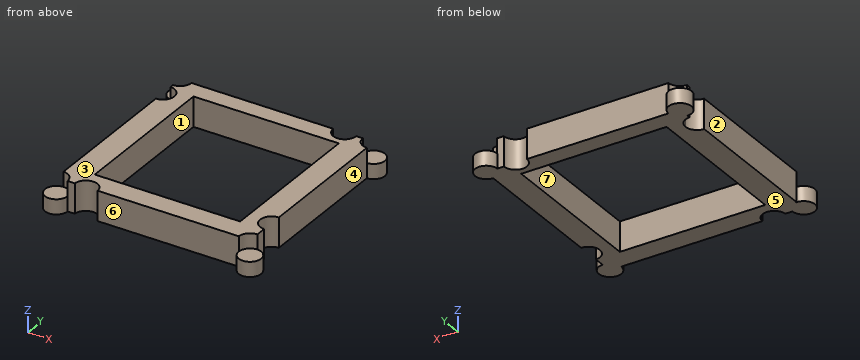
```python
from build123d import *

# Parameters (mm, degrees)
F0_W     = 130.696968
F0_H     = 130.696968
F1_DEPTH = 20
F3_DEPTH = 20
F4_W     = 97.922124
F4_H     = 104.10668
F5_DEPTH = 25
F6_R     = 7.559223
F6_R_2   = 7.71768
F7_DEPTH = 10


with BuildPart() as f1:
    # F0 (on Top) → F1 (new body)
    with BuildSketch(Plane.XY):
        Rectangle(F0_W, F0_H)
    extrude(amount=F1_DEPTH)

    # F2 (on Top) → F3 (cut)
    with BuildSketch(Plane.XY):
        with BuildLine():
            Line((65.463071, -65.384018), (65.463071, -73.302153))
            ThreePointArc((65.463071, -73.302153), (70.877053, -70.99904), (73.111326, -65.556288))
            ThreePointArc((73.111326, -65.556288), (65.450978, -57.810279), (57.620266, -65.384018))
            Line((57.620266, -65.384018), (65.463071, -65.384018))
        make_face()
        with BuildLine():
            ThreePointArc((65.266604, -73.302153), (65.364838, -73.302776), (65.463071, -73.302153))
            Line((65.463071, -73.302153), (65.266604, -73.302153))
        make_face()
        with BuildLine():
            Line((-43.278281, -73.302153), (65.266604, -73.302153))
            ThreePointArc((65.266604, -73.302153), (59.79244, -70.937409), (57.620266, -65.384018))
            Line((57.620266, -65.384018), (-37.424044, -65.384018))
            ThreePointArc((-37.424044, -65.384018), (-37.416151, -65.585784), (-37.413519, -65.787688))
            ThreePointArc((-37.413519, -65.787688), (-39.053255, -70.553782), (-43.278281, -73.302153))
        make_face()
        with BuildLine():
            ThreePointArc((-47.041733, -73.302153), (-45.160007, -73.534176), (-43.278281, -73.302153))
            Line((-43.278281, -73.302153), (-47.041733, -73.302153))
        make_face()
        with BuildLine():
            Line((-52.89597, -65.384018), (-37.424044, -65.384018))
            ThreePointArc((-37.424044, -65.384018), (-45.160007, -58.0412), (-52.89597, -65.384018))
        make_face()
        with BuildLine():
            Line((-52.89597, -73.302153), (-47.041733, -73.302153))
            ThreePointArc((-47.041733, -73.302153), (-51.140461, -70.711329), (-52.89597, -66.191358))
            Line((-52.89597, -66.191358), (-52.89597, -73.302153))
        make_face()
        with BuildLine():
            Line((-52.89597, -66.191358), (-52.89597, -65.384018))
            ThreePointArc((-52.89597, -65.384018), (-52.906495, -65.787688), (-52.89597, -66.191358))
        make_face()
        with BuildLine():
            ThreePointArc((-73.248961, -65.359679), (-65.60328, -73.302152), (-57.75848, -65.556288))
            ThreePointArc((-57.75848, -65.556288), (-60.027374, -60.078694), (-65.504968, -57.8098))
            Line((-65.504968, -57.8098), (-65.504968, -65.365049))
            Line((-65.504968, -65.365049), (-73.248961, -65.365049))
            Line((-73.248961, -65.365049), (-73.248961, -65.359679))
        make_face()
        with BuildLine():
            ThreePointArc((-73.248961, -65.359679), (-70.912604, -60.009617), (-65.504968, -57.8098))
            Line((-65.504968, -57.8098), (-65.504968, 39.620381))
            ThreePointArc((-65.504968, 39.620381), (-70.912604, 41.820198), (-73.248961, 47.17026))
            Line((-73.248961, 47.17026), (-73.248961, -65.359679))
        make_face()
        with BuildLine():
            Line((-65.504968, 54.955278), (-65.504968, 39.620381))
            ThreePointArc((-65.504968, 39.620381), (-60.027374, 41.889275), (-57.75848, 47.366869))
            ThreePointArc((-57.75848, 47.366869), (-60.608689, 53.369745), (-67.061929, 54.955278))
            Line((-67.061929, 54.955278), (-65.504968, 54.955278))
        make_face()
        with BuildLine():
            ThreePointArc((-73.248961, 47.563477), (-73.251456, 47.366869), (-73.248961, 47.17026))
            Line((-73.248961, 47.17026), (-73.248961, 47.563477))
        make_face()
        with BuildLine():
            Line((-73.248961, 54.955278), (-73.248961, 47.563477))
            ThreePointArc((-73.248961, 47.563477), (-71.445222, 52.338937), (-67.061929, 54.955278))
            Line((-67.061929, 54.955278), (-73.248961, 54.955278))
        make_face()
        with BuildLine():
            ThreePointArc((-64.895208, 73.134162), (-71.194062, 60.154116), (-57.75848, 65.411709))
            Line((-57.75848, 65.411709), (-65.504968, 65.411709))
            Line((-65.504968, 65.411709), (-65.504968, 73.134162))
            Line((-65.504968, 73.134162), (-64.895208, 73.134162))
        make_face()
        with BuildLine():
            ThreePointArc((-64.895208, 73.134162), (-59.815874, 70.669303), (-57.75848, 65.411709))
            Line((-57.75848, 65.411709), (37.749253, 65.411709))
            ThreePointArc((37.749253, 65.411709), (45.477167, 73.012411), (53.20508, 65.411709))
            Line((53.20508, 65.411709), (53.20508, 73.134162))
            Line((53.20508, 73.134162), (-64.895208, 73.134162))
        make_face()
        with BuildLine():
            Line((53.20508, 65.411709), (37.749253, 65.411709))
            ThreePointArc((37.749253, 65.411709), (45.413026, 57.554721), (53.206145, 65.283433))
            ThreePointArc((53.206145, 65.283433), (53.205879, 65.347573), (53.20508, 65.411709))
        make_face()
        with BuildLine():
            Line((73.154315, 65.283433), (73.170148, 65.283433))
            ThreePointArc((73.170148, 65.283433), (59.946066, 70.761027), (65.42366, 57.536945))
            Line((65.42366, 57.536945), (65.42366, 65.283433))
            Line((65.42366, 65.283433), (73.154315, 65.283433))
        make_face()
        with BuildLine():
            Line((73.265217, 65.283433), (73.170148, 65.283433))
            ThreePointArc((73.170148, 65.283433), (70.901254, 59.805838), (65.42366, 57.536945))
            Line((65.42366, 57.536945), (65.42366, -35.264168))
            ThreePointArc((65.42366, -35.264168), (70.901254, -37.533062), (73.170148, -43.010656))
            ThreePointArc((73.170148, -43.010656), (71.089749, -48.293033), (65.965977, -50.738137))
            Line((65.965977, -50.738137), (73.265217, -50.738137))
            Line((73.265217, -50.738137), (73.265217, 65.283433))
        make_face()
        with BuildLine():
            Line((65.42366, -50.738137), (65.42366, -35.264168))
            ThreePointArc((65.42366, -35.264168), (57.681925, -43.281981), (65.965977, -50.738137))
            Line((65.965977, -50.738137), (65.42366, -50.738137))
        make_face()
    extrude(amount=F3_DEPTH, mode=Mode.SUBTRACT)

    # F4 (on Top) → F5 (cut)
    with BuildSketch(Plane.XY):
        with Locations((0.309229, 1.133837)):
            Rectangle(F4_W, F4_H)
    extrude(amount=F5_DEPTH, mode=Mode.SUBTRACT)

    # F6 (on Top) → F7 (join)
    with BuildSketch(Plane.XY):
        with Locations((-65.319784, -65.393053)):
            Circle(F6_R)
        with Locations((65.150194, -65.393053)):
            Circle(F6_R)
        with Locations((-65.368432, 65.110195)):
            Circle(F6_R_2)
        with Locations((65.150194, 65.110195)):
            Circle(F6_R)
    extrude(amount=F7_DEPTH)


solid = f1.part
```
The listing builds one solid part. Answer for the finished solid, in the listing's coordinates (mm). Face numbers are marked on the shaded views. A direction names the side the tool comes from. Coordinates: 2 decimals unless noted, no trailing zeros. Loops run counter-clockwise (first coordinate to the right, second up) from the corner with the lowest first, then second, coordinate; pieces in that order, holes last. Notation, with made-up numbers: (79.25, 46) - (91.25, 46) arc R15 cw to (91.25, 68) - close; hole circle Ø8 at (53.25, 17). An arc over 180 degrees is marked (long way). Use a Markdown table: item, result. Add a question column.
1) The part is cut by section B-B, the plane z = 18. Give the vertices of the cut face in (x, y), and give its area (3 significant figures).
2) The part is cut by section C-C, the plane x = 3. Give the vertices of the cut face in (y, z).
3) For the marked faces 1, 2, 3 and 4, determine the directions among +Z, -Z, +X, -X, +Y, -Y from which every point of the face is accessible in a straight line to the end or side of a thin tool.
4) The part is cut by section D-D, the plane z = 2. Give the vertices of the cut face in (x, y).
5) The part is cut by section A-A, the plane y = 6. Give the vertices of the cut face in (x, z), and give its area (3 significant figures).
6) The mould has two halves that part along Y. Classify the marked faces 5, 6 and 7: released by +Y, released by -Y, zero draft, split by the parting line, or undercut.
7) Find the intervals of material crossed by line 1 (X direction, y = 9, z = 15.75); line 2 (Y direction, x = -35, z = 8.25); line 3 (X direction, y = -59, z = 12.5), in increasing order.
8) Given pin 1 (12 mm diameter, centred on x = 68.5, y = 63.5, fed in from +Z); pin 2 (10 mm diameter, centred on y = -20, z = 13, fed in from +X); pin 3 (6 mm diameter, centred on x = -11, z = 7.5, fed in from -Y), each flat-ended and moving along its own axis, determine where each tip first touches the part or whether it passes through.
Here are the results:
| question | item | result |
|---|---|---|
| 1 | outline | (-65.35, -57.81) arc R7.75 cw to (-57.76, -65.35) - (-52.89, -65.35) arc R7.75 cw to (-37.43, -65.35) - (57.62, -65.35) arc R7.75 cw to (65.35, -57.81) - (65.35, -50.76) arc R7.75 cw to (65.35, -35.26) - (65.35, 57.54) arc R7.75 cw to (57.68, 65.35) - (53.21, 65.35) arc R7.72 cw to (53.21, 65.28) arc R7.73 cw (long way) to (37.75, 65.35) - (-57.76, 65.35) arc R7.75 cw to (-65.35, 57.67) - (-65.35, 55.11) arc R7.75 cw to (-57.76, 47.37) arc R7.75 cw to (-65.35, 39.62) - close; hole (-48.65, -50.92) - (49.27, -50.92) - (49.27, 53.19) - (-48.65, 53.19) - close |
| 1 | area | 6,340 mm^2 |
| 2 | outline | (-65.35, 0) - (-50.92, 0) - (-50.92, 20) - (-65.35, 20) - close; (53.19, 0) - (65.35, 0) - (65.35, 20) - (53.19, 20) - close |
| 3 | face 1 | +Z, -Z |
| 3 | face 2 | +Z, -Z, -X |
| 3 | face 3 | +Z, +X, -X, +Y, -Y |
| 3 | face 4 | +Z, -Z, +X |
| 4 | outline | (-65.35, -57.81) arc R7.75 cw to (-64.35, -57.9) arc R7.56 ccw (long way) to (-57.76, -65.35) - (-52.89, -65.35) arc R7.75 cw to (-37.43, -65.35) - (57.59, -65.35) arc R7.56 ccw (long way) to (64.36, -57.88) arc R7.75 cw to (65.35, -57.81) - (65.35, -50.76) arc R7.75 cw to (65.35, -35.26) - (65.35, 57.54) arc R7.75 cw to (64.89, 57.56) arc R7.56 ccw (long way) to (57.59, 65.35) - (53.21, 65.35) arc R7.72 cw to (53.21, 65.28) arc R7.73 cw (long way) to (37.75, 65.35) - (-57.65, 65.35) arc R7.72 ccw (long way) to (-65.35, 57.39) - (-65.35, 55.11) arc R7.75 cw to (-57.76, 47.37) arc R7.75 cw to (-65.35, 39.62) - close; hole (-48.65, -50.92) - (49.27, -50.92) - (49.27, 53.19) - (-48.65, 53.19) - close |
| 5 | outline | (-65.35, 0) - (-48.65, 0) - (-48.65, 20) - (-65.35, 20) - close; (49.27, 0) - (65.35, 0) - (65.35, 20) - (49.27, 20) - close |
| 5 | area | 655 mm^2 |
| 6 | face 5 | zero draft |
| 6 | face 6 | released by -Y |
| 6 | face 7 | undercut |
| 7 | line 1 | x = -65.35 to -48.65, 49.27 to 65.35 |
| 7 | line 2 | y = -65.35 to -50.92, 53.19 to 65.35 |
| 7 | line 3 | x = -61.38 to -48.89, -41.43 to 61.24 |
| 8 | pin 1 | stops at z = 10 |
| 8 | pin 2 | stops at x = 65.35 |
| 8 | pin 3 | stops at y = -65.35 |
